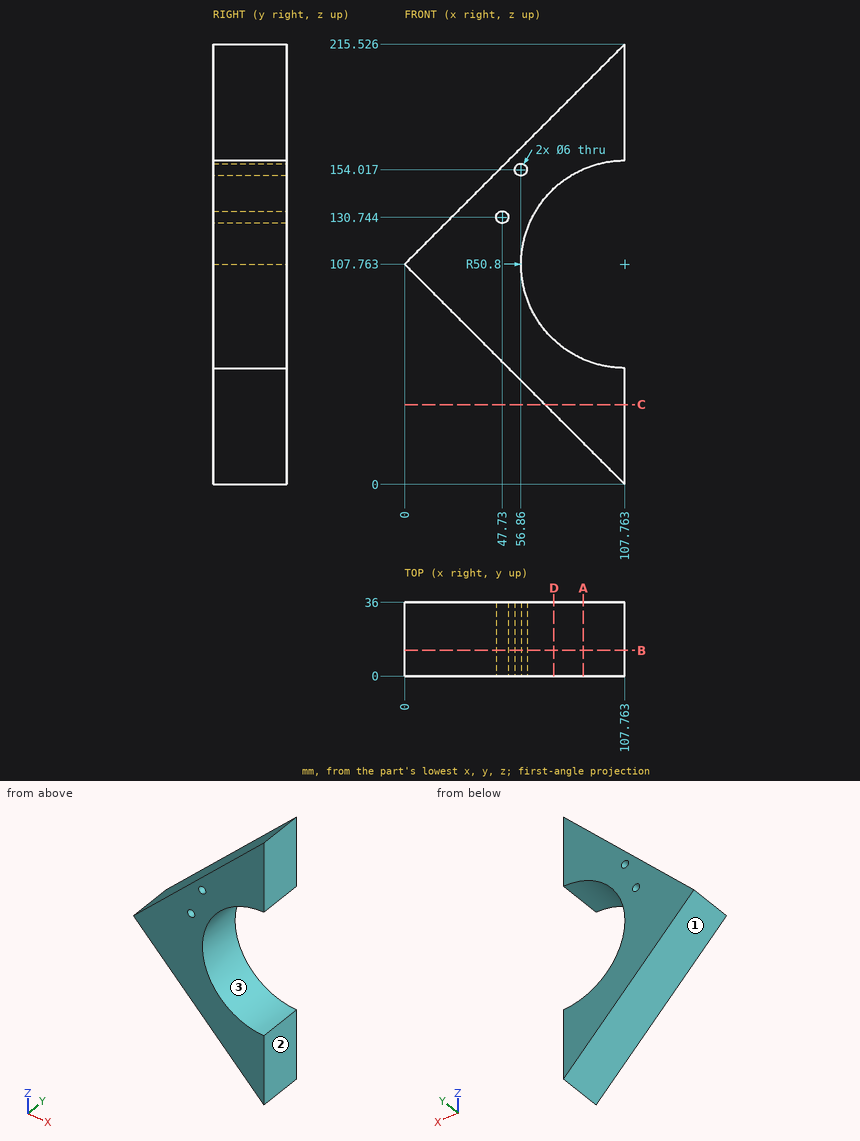
Source: three-view drawing plus pictorial views. Frame: mm from the lowest corner of the part. Coordinates: 2 decimals unless noted, no trailing zeros. Loops run counter-clockwise (first coordinate to the right, second up) from the corner with the lowest first, then second, coordinate; pieces in that order, holes last. Notation, with made-up numbers: M 81,61.5 L 103,61.5 A32 ccw 103,99.5 Z; hole C 39,84.5 d7. An arc over 180 degrees is marked long. Use CSV: the item, a comma, the result in double quotes.
(1) Contact query for flat-ended pins moving along their axis: pin 1 (4 mm diameter, centred on y = 24, z = 137, fed in from -X) (1 decimal); pin 2 (12 mm diameter, centred on x = 88, y = 31.5, fed in from -Z) (1 decimal); pin 3 (10 mm diameter, centred on x = 73.5, y = 20.5, fed in from +Z) (1 decimal); pin 4 (3.5 mm diameter, centred on x = 56.86, z = 154.02, fed in from +Y). Output: stop coordinate, or through.
Answers follow:
pin 1,"x = 27.2"
pin 2,"z = 13.8"
pin 3,"z = 186.3"
pin 4,"through"
(2) Cut plane C-C on z = 39. Return loops of the section in (x, y).
Answers follow:
outline,"M 68.76,0 L 107.76,0 L 107.76,36 L 68.76,36 Z"
(3) Draft query along Z for the marked faces 1, 2 and 3. Return one class per face: pulls with the +Z half, pulls with the -Z half, needs draft (parallel to the pull), parting line crosses it, or undercut.
Answers follow:
face 1,"pulls with the -Z half"
face 2,"needs draft"
face 3,"undercut"
(4) Cut plane D-D on x = 73. Return loops of the section in (y, z) (1 decimal), and give its area (3 significant figures).
Answers follow:
outline,"M 0,34.8 L 36,34.8 L 36,70.7 L 0,70.7 Z; M 0,144.8 L 36,144.8 L 36,180.8 L 0,180.8 Z"
area,"2,590 mm²"
(5) Line query: line 1 (Z direction, x = 67.5, y = 31) (1 decimal); line 2 (Z direction, x = 61, y = 13) (1 decimal); line 3 (X direction, y = 8.5, z = 164) (1 decimal). Output: solid intervals per line, ascending. Write a range as [from, to].
Answers follow:
line 1,"[40.3, 76.8], [138.7, 175.3]"
line 2,"[46.8, 87.9], [127.6, 168.8]"
line 3,"[56.2, 107.8]"
(6) Cut plane A-A on x = 87.5. Return loops of the section in (y, z).
Answers follow:
outline,"M 0,20.26 L 36,20.26 L 36,61.18 L 0,61.18 Z; M 0,154.35 L 36,154.35 L 36,195.26 L 0,195.26 Z"
(7) Cut plane B-B on y = 12.5. Return loops of the section in (x, z) (1 decimal), and give its area (3 significant figures).
Answers follow:
outline,"M 0,107.8 L 107.8,0 L 107.8,57 A50.8 cw 107.8,158.6 L 107.8,215.5 Z; hole C 47.7,130.7 d6; hole C 56.9,154 d6"
area,"7,500 mm²"
